from build123d import *

# Parameters (mm, degrees)
F1_DEPTH = 25
F2_SIZE  = 0.5
F4_DEPTH = 4
F5_R     = 1


with BuildPart() as f1:
    # F0 (on Top) → F1 (new body)
    with BuildSketch(Plane.XY):
        Polygon((-32.75, 4), (-32.75, -7.25), (7.25, -7.25), (7.25, 32.75), (-4, 32.75), (-4, 4), align=None)
        with BuildLine():
            Line((0, 4), (0, 28.75))
            Line((0, 28.75), (3.25, 28.75))
            Line((3.25, 28.75), (3.25, -3.25))
            Line((3.25, -3.25), (-28.75, -3.25))
            Line((-28.75, -3.25), (-28.75, 0))
            Line((-28.75, 0), (-4, 0))
            ThreePointArc((-4, 0), (-1.171573, 1.171573), (0, 4))
        make_face(mode=Mode.SUBTRACT)
    extrude(amount=F1_DEPTH)

    # F2
    f2_edges = [f1.edges().sort_by_distance(p)[0] for p in [
        (-32.75, -1.625, 25),
        (-12.75, -7.25, 25),
        (7.25, 12.75, 25),
        (1.625, 32.75, 25),
        (-4, 18.375, 25),
        (-18.375, 4, 25),
        (0, 16.375, 25),
        (1.625, 28.75, 25),
        (3.25, 12.75, 25),
        (-12.75, -3.25, 25),
        (-28.75, -1.625, 25),
        (-16.375, 0, 25),
        (-1.171573, 1.171573, 25),
    ]]
    chamfer(f2_edges, length=F2_SIZE)

    # F3 (on face) → F4 (join)
    with BuildSketch(Plane(origin=(0, 0, 0), x_dir=(1, 0, 0), z_dir=(0, 0, -1))):
        Polygon((7.25, 7.25), (-32.75, 7.25), (-32.75, -4), (-4, -4), (-4, -32.75), (7.25, -32.75), align=None)
    extrude(amount=F4_DEPTH)

    # F5
    f5_edges = [f1.edges().sort_by_distance(p)[0] for p in [
        (-12.75, -7.25, -4),
        (-32.75, -1.625, -4),
        (-18.375, 4, -4),
        (-4, 18.375, -4),
        (1.625, 32.75, -4),
        (7.25, 12.75, -4),
    ]]
    fillet(f5_edges, radius=F5_R)


solid = f1.part
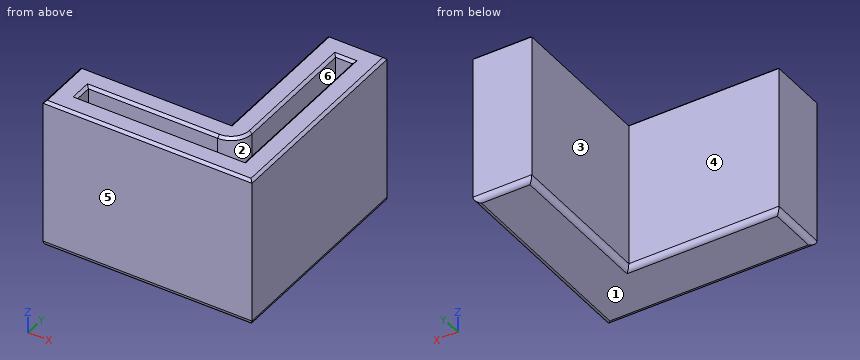
Part model, mm, in its own coordinate system. Face numbers are marked on the shaded views. A direction names the side the tool comes from. Coordinates: 2 decimals unless noted, no trailing zeros. Order: outer loops, then holes, each group sorted by start corner. A loop starts at its lowest first (then second) coordinate and runs counter-clockwise, first axis right, second up.
(1) Slice it at C-C, the plane y = 14. Write the cut outline in (x, z), and give its area (3 significant figures).
Check sheet entries:
outline: (-4, -3) arc R1 ccw to (-3, -4) - (6.25, -4) arc R1 ccw to (7.25, -3) - (7.25, 24.5) - (6.75, 25) - (3.75, 25) - (3.25, 24.5) - (3.25, 0) - (0, 0) - (0, 24.5) - (-0.5, 25) - (-3.5, 25) - (-4, 24.5) - close
area: 244 mm2
(2) Pin check, flat tips, straight feed: pin 1 Ø8 at (y, z) = (14.5, 9) entering from -X; pin 2 Ø16 at (x, y) = (-18.5, 20) entering from +Z; pin 3 Ø12 at (x, z) = (-12, 15) entering from +Y. Stop position of each tip, or through.
Check sheet entries:
pin 1: stops at x = -4
pin 2: passes through
pin 3: stops at y = 4
(3) Tool access for the marked faces 1 and 2: list every direction of +Z, -Z, +X, -X, +Y, -Y with a clear straight run to the whole face (end or side of a thin tool).
Check sheet entries:
face 1: -Z, +X, -X, +Y, -Y
face 2: +Z
(4) Slice it at B-B, the plane x = -22. Write the cut outline in (y, z).
Check sheet entries:
outline: (-7.25, -3) arc R1 ccw to (-6.25, -4) - (3, -4) arc R1 ccw to (4, -3) - (4, 24.5) - (3.5, 25) - (0.5, 25) - (0, 24.5) - (0, 0) - (-3.25, 0) - (-3.25, 24.5) - (-3.75, 25) - (-6.75, 25) - (-7.25, 24.5) - close
(5) Probe L1, parallel to Y at x = -20, z = 9; L2, parallel to X at y = 23.5, z = 1.75. List the from-to ranges inside material, lowest first.
Check sheet entries:
L1: y = -7.25 to -3.25, 0 to 4
L2: x = -4 to 0, 3.25 to 7.25
(6) Pull direction Y, two halves, no side cores. Call the marked faces 3, 4, 5 and 6: pulls with the +Y half, pulls with the -Y half, needs draft (parallel to the pull), parting line crosses it, or undercut.
Check sheet entries:
face 3: needs draft
face 4: pulls with the +Y half
face 5: pulls with the -Y half
face 6: undercut
(7) Slice it at A-A, the plane z = 15.75. Write the cut outline in (x, y), and give its area (3 significant figures).
Check sheet entries:
outline: (-32.75, -7.25) - (7.25, -7.25) - (7.25, 32.75) - (-4, 32.75) - (-4, 4) - (-32.75, 4) - close; hole (-28.75, -3.25) - (3.25, -3.25) - (3.25, 28.75) - (0, 28.75) - (0, 4) arc R4 cw to (-4, 0) - (-28.75, 0) - close
area: 573 mm2
